Geometry check sheet. Reference: the model listing, model coordinates, mm. A direction names the side the tool comes from. Coordinates: 2 decimals unless noted, no trailing zeros. Write each loop counter-clockwise with the first axis right and the second up, starting at its lowest first coordinate (ties: lowest second). Pieces come first, ordered by that corner, then holes. Notation, with made-up numbers: (0.5, -10.5) -> (30.5, -10.5) arc R21 ccw to (30.5, 3.5) -> close; hole circle Ø9 at (31.25, -17.5). An arc over 180 degrees is marked (long way). Answer as CSV lines item,"result".
```python
from build123d import *

# Parameters (mm, degrees)
F0_R           = 8.95
F1_DEPTH       = 8
F2_R           = 8.95
F2_R_2         = 7.55
F3_DEPTH       = 2.8
F5_DEPTH       = 13.2
F6_R           = 1
F8_DEPTH       = 7.7
F9_W           = 1.29
F9_H           = 7.7
F10_DEPTH      = 1.5
F10_DEPTH_BACK = 8


with BuildPart() as f1:
    # F0 (on Top) → F1 (new body)
    with BuildSketch(Plane.XY):
        Circle(F0_R)
    extrude(amount=F1_DEPTH)

    # F2 (on face) → F3 (join)
    with BuildSketch(Plane.XY.offset(8)):
        Circle(F2_R)
        Circle(F2_R_2, mode=Mode.SUBTRACT)
    extrude(amount=F3_DEPTH)

    # F4 (on face) → F5 (join)
    with BuildSketch(Plane.XY.offset(8)):
        with BuildLine():
            ThreePointArc((-4.1, -3.0331501776), (1.5968719423, -4.8435524153), (5.1, 0))
            ThreePointArc((5.1, 0), (1.5968719423, 4.8435524153), (-4.1, 3.0331501776))
            Line((-4.1, 3.0331501776), (-4.1, -3.0331501776))
        make_face()
    extrude(amount=F5_DEPTH)

    # F6
    f6_edges = [f1.edges().sort_by_distance(p)[0] for p in [
        (-8.95, 0, 0),
    ]]
    fillet(f6_edges, radius=F6_R)

    # F7 (on face) → F8 (cut)
    with BuildSketch(Plane.XY.offset(21.2)):
        with BuildLine():
            Line((-2.9, 2.6076809621), (-2.9, -2.6076809621))
            ThreePointArc((-2.9, -2.6076809621), (3.9, 0), (-2.9, 2.6076809621))
        make_face()
    extrude(amount=-F8_DEPTH, mode=Mode.SUBTRACT)

    # F9 (on face) → F10 (cut, two sides)
    with BuildSketch(Plane.YZ.offset(-2.9)) as f10_sk:
        with Locations((-0.0373190379, 17.35)):
            Rectangle(F9_W, F9_H)
    extrude(amount=-F10_DEPTH, mode=Mode.SUBTRACT)
    extrude(f10_sk.sketch, amount=F10_DEPTH_BACK, mode=Mode.SUBTRACT)


solid = f1.part
```
Item 1: Cross-section at A-A, the plane z = 8.75. Record the cut outline in (x, y), plus the area to 3 significant figures.
Responses:
outline,"circle Ø17.9 at (0, 0); (-4.1, -3.03) arc R5.1 ccw (long way) to (-4.1, 3.03) -> close; hole circle Ø15.1 at (0, 0)"
area,"150 mm2"
Item 2: Release check for a two-part mould opening along Y. For faces 4 (the flat face through (0, 0, 0)), 5 (the cylindrical face through (1.012, -3.766, 17.404)), 6 (the cylindrical face through (-7.1, -5.45, 5.83)) record: +Y half, -Y half, draft (parallel to the pull), parting line (faces both ways), or undercut.
Responses:
face 4,"draft"
face 5,"undercut"
face 6,"parting line"
Item 3: Depth check by flat-ended pin: pin 1 Ø1 at (y, z) = (-3, 3.5) entering from +X; pin 2 Ø1 at (x, z) = (-3.5, 16) entering from +Y; pin 3 Ø1 at (x, z) = (4.5, 17) entering from +Y; pin 4 Ø1 at (y, z) = (6.5, 18.5) entering from -X. Enter the tip coordinate at first touch or a pass-through.
Responses:
pin 1,"stops at x = 8.59"
pin 2,"stops at y = 4.12"
pin 3,"stops at y = 3.16"
pin 4,"passes through"
Item 4: Cross-section at B-B, the plane z = 15.5. Record the cut outline in (x, y).
Responses:
outline,"(-4.1, -3.03) arc R5.1 ccw to (5.05, -0.68) -> (3.84, -0.68) arc R3.9 cw to (-2.9, -2.61) -> (-2.9, -0.68) -> (-4.1, -0.68) -> close; (-4.1, 0.61) -> (-2.9, 0.61) -> (-2.9, 2.61) arc R3.9 cw to (3.85, 0.61) -> (5.06, 0.61) arc R5.1 ccw to (-4.1, 3.03) -> close"
Item 5: Set-up check for faces 1 (the flat face through (-1, 4, 21.2)), 2 (the flat face through (-3.5, -0.682, 17.3)), 3 (the cylindrical face through (1.17, 3.72, 17.4)): record each of +Z, -Z, +X, -X, +Y, -Y from which the full face is reachable in a straight line by a thin tool's end or side.
Responses:
face 1,"+Z, +X, -X, +Y, -Y"
face 2,"+Z, +X, -X"
face 3,"+Z"
Item 6: Thickness scan on probe 1 along Y at (x, z) = (0, 9.9); probe 2 along Z at (x, y) = (2.5, 5.5); probe 3 along Z at (x, y) = (5, -6.25). Record the ranges inside material, lowest first.
Responses:
probe 1,"y = -8.95 to -7.55, -5.1 to 5.1, 7.55 to 8.95"
probe 2,"z = 0 to 8"
probe 3,"z = 0 to 10.8"
Item 7: Cross-section at C-C, the plane x = 0. Record the cut outline in (y, z), plus the area to 3 significant figures.
Responses:
outline,"(-8.95, 1) arc R1 ccw to (-7.95, 0) -> (7.95, 0) arc R1 ccw to (8.95, 1) -> (8.95, 10.8) -> (7.55, 10.8) -> (7.55, 8) -> (5.1, 8) -> (5.1, 21.2) -> (3.9, 21.2) -> (3.9, 13.5) -> (-3.9, 13.5) -> (-3.9, 21.2) -> (-5.1, 21.2) -> (-5.1, 8) -> (-7.55, 8) -> (-7.55, 10.8) -> (-8.95, 10.8) -> close"
area,"225 mm2"
Item 8: Cross-section at D-D, the plane z = 4.5. Record the cut outline in (x, y), plus the area to 3 significant figures.
Responses:
outline,"circle Ø17.9 at (0, 0)"
area,"252 mm2"
